Source: CAD feature listing. Evaluate the final solid. Frame: model axes, mm. Face numbers are marked on the shaded views. Coordinates: 2 decimals unless noted, no trailing zeros. Order: outer loops, then holes, each group sorted by start corner. A loop starts at its lowest first (then second) coordinate and runs counter-clockwise, first axis right, second up. Notation, with made-up numbers: (-5, -2.75) - (16, -2.75) arc R12 cw to (16, 20.25) - close; hole circle Ø10 at (19, -18.75). An arc over 180 degrees is marked (long way). One line per question, with ' | ' between items. Start each with the question number.
(1) Contact query for flat-ended pins moving along their axis: P1, Ø25, axis at x = 126, y = 18.5, coming from the +Z side; P2, Ø12, axis at x = 173, z = 40.5, coming from the +Y side; P3, Ø1, axis at x = 154.5, z = 49, coming from the -Y side; P4, Ø7.5, axis at y = 0, z = 0, coming from the +X side. Output: stop coordinate, or through.
(2) Section A-A (y = 0). Return the cut outline in (x, z) (3 decimals).
(3) Section D-D (y = 64). Return the cut outline in (x, z).
(4) Draft query along Y for the marked faces 1, 2, 3 and 4. Return one class per face: +Y half, -Y half, draft (parallel to the pull), parting line (faces both ways), or undercut.
(5) Section C-C (z = 41). Return the cut outline in (x, y).
(6) Line query: line 1 along Z through (x, y) = (121, 0) (3 decimals); line 2 along Y through (x, z) = (192, 4.5); line 3 along Y through (x, z) = (59, 47.5). Output: solid intervals per line, ascending.
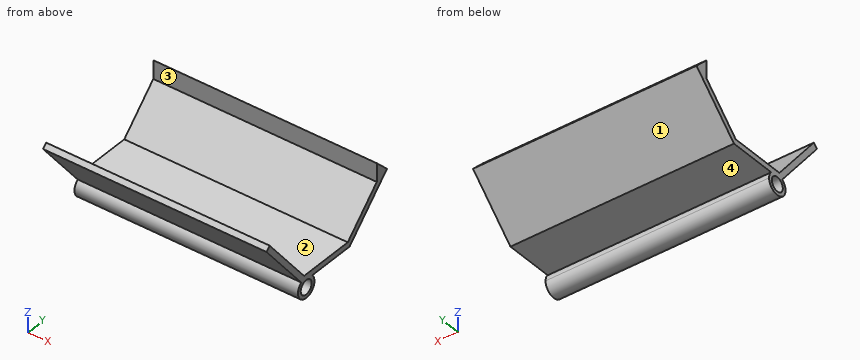
from build123d import *

# Parameters (mm, degrees)
F0_R     = 6.35
F1_DEPTH = 200


with BuildPart() as f1:
    # F0 (on Right) → F1 (new body)
    with BuildSketch(Plane.YZ):
        with BuildLine():
            ThreePointArc((-5.7829078209, 7.568593141), (-4.2215771937, -8.5383787101), (9.525, 0))
            ThreePointArc((9.525, 0), (8.8822194716, 3.4397386904), (7.0406320718, 6.4152260311))
            Line((7.0406320718, 6.4152260311), (-4.86379717, 6.4152260311))
            Line((-4.86379717, 6.4152260311), (-5.7829078209, 7.568593141))
        make_face()
        Circle(F0_R, mode=Mode.SUBTRACT)
        with BuildLine():
            Line((-4.86379717, 6.4152260311), (7.0406320718, 6.4152260311))
            ThreePointArc((7.0406320718, 6.4152260311), (0.8532476167, 9.4867061462), (-5.7829078209, 7.568593141))
            Line((-5.7829078209, 7.568593141), (-4.86379717, 6.4152260311))
        make_face()
        with BuildLine():
            ThreePointArc((-5.7829078209, 7.568593141), (0.8532476167, 9.4867061462), (7.0406320718, 6.4152260311))
            Line((7.0406320718, 6.4152260311), (50.0992612617, 6.4152260311))
            Line((50.0992612617, 6.4152260311), (93.3420076617, 49.6579724311))
            Line((93.3420076617, 49.6579724311), (85.4284786876, 57.5715014053))
            Line((85.4284786876, 57.5715014053), (81.5560158427, 61.4152260311))
            Line((81.5560158427, 61.4152260311), (81.5560158427, 44.943048424))
            Line((81.5560158427, 44.943048424), (48.0281934499, 11.4152260311))
            Line((48.0281934499, 11.4152260311), (-2.454831837, 11.4152260311))
            Line((-2.454831837, 11.4152260311), (-42.2995024128, 61.4152260311))
            Line((-42.2995024128, 61.4152260311), (-45.8575500686, 57.8571783753))
            Line((-45.8575500686, 57.8571783753), (-5.7829078209, 7.568593141))
        make_face()
    extrude(amount=F1_DEPTH)


solid = f1.part
Response values:
1) P1: stops at z = 11.42 | P2: stops at y = 90.18 | P3: stops at y = -39.2 | P4: passes through
2) outline: (0, -9.525) - (200, -9.525) - (200, -6.35) - (0, -6.35) - close; (0, 6.35) - (200, 6.35) - (200, 11.415) - (0, 11.415) - close
3) outline: (0, 20.32) - (200, 20.32) - (200, 27.39) - (0, 27.39) - close
4) face 1: +Y half | face 2: undercut | face 3: undercut | face 4: draft
5) outline: (0, -32.42) - (200, -32.42) - (200, -26.03) - (0, -26.03) - close; (0, 77.61) - (200, 77.61) - (200, 84.68) - (0, 84.68) - close
6) line 1: z = -9.525 to -6.35, 6.35 to 11.415 | line 2: y = -8.39 to -4.48, 4.48 to 8.39 | line 3: y = -37.6 to -31.21, 81.56 to 91.18
